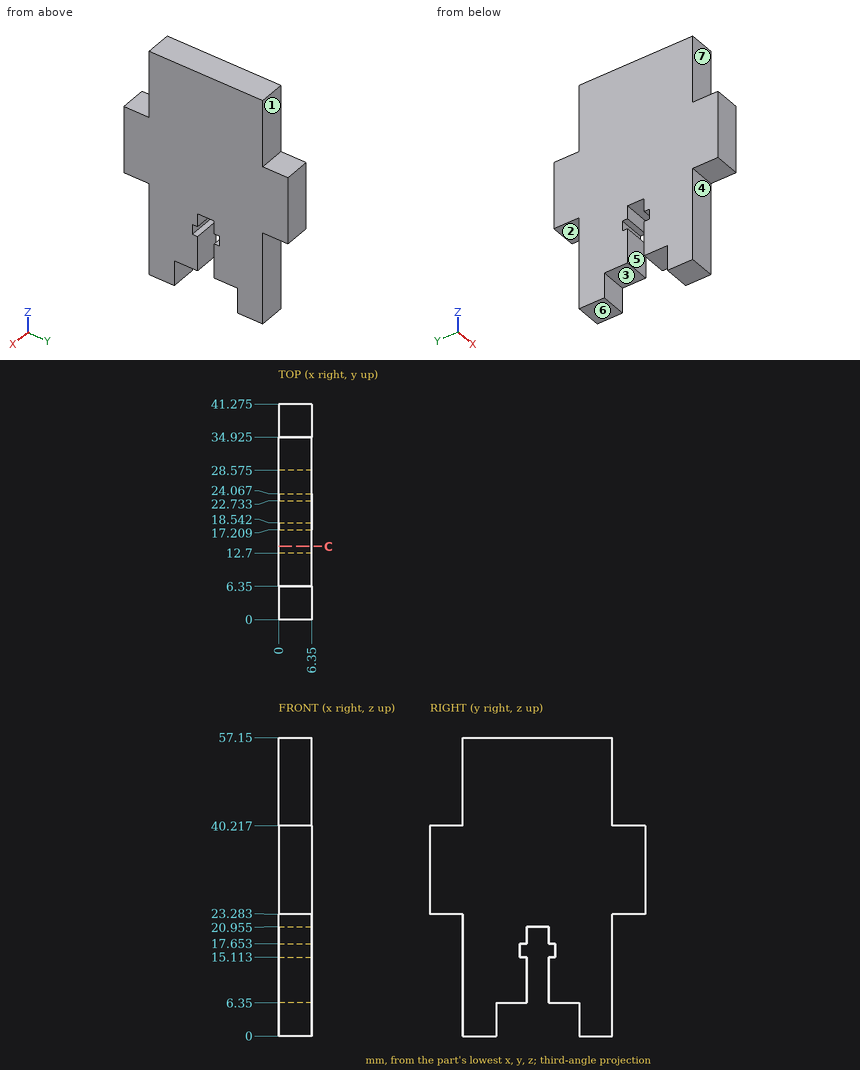
Could you check a few things on this drawing? It's one solid part, dimensions in mm from its lowest x, y, z. A direction names the side the tool comes from. Give positions to 0.01 mm unless a question says otherwise; leave off trailing zeros. Write each loop counter-clockwise with the first axis right and the second up, starting at its lowest first coordinate (ties: lowest second). Pieces come first, ordered by that corner, then holes. Notation, with made-up numbers: M -5.5,47 L 31.5,47 A19 cw 31.5,64 Z; hole C -20.75,67.5 d5. An arc over 180 degrees is marked long. Put each result on its own line as item: value. Start each with the question number.
Item 1: I need wall thicknesses on L1, parallel to Z at x = 3.25, y = 18; L2, parallel to Z at x = 1, y = 2.5; L3, parallel to Z at x = 4.5, y = 28. Which ranges of each line are inside material? Lowest first, please. Write a range as from..to.
Item 2: On a 3-axis mill with a long thin cutter (end or side, diameter ignored), from which of +Z, -Z, +X, -X, +Y, -Y can I reach the whole of each face in a straight line? I mean the marked faces 1, 2, 3 and 4. Say none if no direction works.
Item 3: If we section it at C-C, the plane y = 14: Write out the boundary of the cut face in (x, z).
Item 4: Will these pins go through, and if not, where does the flat tip stop? pin 1 (3 mm diameter, centred on x = 4, z = 10.5, fed in from -Y); pin 2 (1.8 mm diameter, centred on x = 4, y = 26, fed in from -Z); pin 3 (2 mm diameter, centred on x = 3.5, z = 16, fed in from +Y) (1 decimal).
Item 5: Thinking about a two-plate mould opening in Y: for the marked faces 5, 6 and 7, which applies, +Y half, -Y half, draft (parallel to the pull), parting line (faces both ways), or undercut?
Values:
1. L1: 6.35..15.11, 17.65..57.15
1. L2: 23.28..40.22
1. L3: 6.35..57.15
2. face 1: +Z, +X, -X, +Y
2. face 2: -Z, +X, -X, +Y
2. face 3: -Z, +X, -X
2. face 4: -Z, +X, -X, -Y
3. outline: M 0,6.35 L 6.35,6.35 L 6.35,57.15 L 0,57.15 Z
4. pin 1: y = 6.35
4. pin 2: z = 6.35
4. pin 3: y = 34.9
5. face 5: undercut
5. face 6: draft
5. face 7: -Y half
